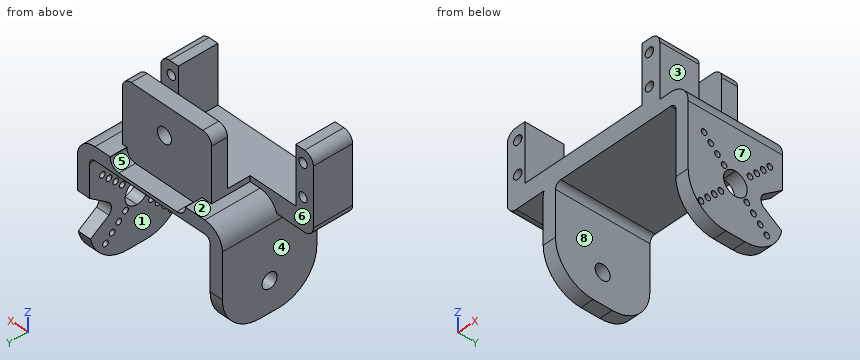
```python
from build123d import *

# Parameters (mm, degrees)
BOSS_EXTRUDE1_DEPTH     = 50
BOSS_EXTRUDE2_DEPTH     = 20.8
SKETCH4_W               = 50.8
SKETCH4_H               = 3
BOSS_EXTRUDE3_DEPTH     = 20.4
BOSS_EXTRUDE4_START     = 32.8
BOSS_EXTRUDE4_OUTLINE_W = 50.8
BOSS_EXTRUDE4_OUTLINE_H = 30.5
BOSS_EXTRUDE4_OUTLINE_R = 4
BOSS_EXTRUDE4_DEPTH     = 8.4
CUT_EXTRUDE1_OUTLINE_R  = 2.4
CUT_EXTRUDE1_DEPTH      = 20.8
FILLET1_R               = 5
FILLET2_R               = 20
SKETCH6_R               = 1.5
CUT_EXTRUDE2_DEPTH      = 28.4
CUT_EXTRUDE3_DEPTH      = 136.4
CUT_EXTRUDE4_DEPTH      = 132.215666798
CUT_EXTRUDE4_DEPTH_BACK = 26.4
CUT_EXTRUDE5_DEPTH      = 8.8


# Read off the part's stored shape, not the designer's step: Boss-Extrude4, Cut-Extrude1
with BuildPart() as part:
    # Sketch1 → Boss-Extrude1 (new body)
    with BuildSketch(Plane(origin=(0, 0, 0), x_dir=(1, 0, 0), z_dir=(0, 1, 0))):
        with BuildLine():
            Line((-56.375697839, 54.197981352), (-56.375697839, 10.497981352))
            ThreePointArc((-56.375697839, 10.497981352), (-53.44676565, 3.42691354), (-46.375697839, 0.497981352))
            Line((-46.375697839, 0.497981352), (16.224302161, 0.497981352))
            ThreePointArc((16.224302161, 0.497981352), (23.295369973, 3.42691354), (26.224302161, 10.497981352))
            Line((26.224302161, 10.497981352), (26.224302161, 64.097981352))
            Line((26.224302161, 64.097981352), (19.224302161, 64.097981352))
            Line((19.224302161, 64.097981352), (19.224302161, 10.497981352))
            ThreePointArc((19.224302161, 10.497981352), (18.345622505, 8.376661008), (16.224302161, 7.497981352))
            Line((16.224302161, 7.497981352), (-46.375697839, 7.497981352))
            ThreePointArc((-46.375697839, 7.497981352), (-48.497018182, 8.376661008), (-49.375697839, 10.497981352))
            Line((-49.375697839, 10.497981352), (-49.375697839, 54.197981352))
            Line((-49.375697839, 54.197981352), (-56.375697839, 54.197981352))
        make_face()
    extrude(amount=BOSS_EXTRUDE1_DEPTH)

    # Sketch2 → Boss-Extrude2 (add)
    with BuildSketch(Plane.XZ):
        with BuildLine():
            Line((-71.775697839, -7.497981352), (-55.915089853, -7.497981352))
            ThreePointArc((-55.915089853, -7.497981352), (-52.291777622, -2.435723603), (-46.375697839, -0.497981352))
            Line((-46.375697839, -0.497981352), (10.024302161, -0.497981352))
            Line((10.024302161, -0.497981352), (10.024302161, 33.002018648))
            Line((10.024302161, 33.002018648), (0.024302161, 33.002018648))
            Line((0.024302161, 33.002018648), (0.024302161, 2.502018648))
            Line((0.024302161, 2.502018648), (-66.775697839, 2.502018648))
            Line((-66.775697839, 2.502018648), (-66.775697839, 33.002018648))
            Line((-66.775697839, 33.002018648), (-76.775697839, 33.002018648))
            Line((-76.775697839, 33.002018648), (-76.775697839, -2.497981352))
            ThreePointArc((-76.775697839, -2.497981352), (-75.311231744, -6.033515257), (-71.775697839, -7.497981352))
        make_face()
    extrude(amount=-BOSS_EXTRUDE2_DEPTH)

    # Sketch4 → Boss-Extrude3 (add)
    with BuildSketch(Plane(origin=(0, 20.8, 0), x_dir=(1, 0, 0), z_dir=(0, 1, 0))):
        with Locations((-15.375697839, -1.002018648)):
            Rectangle(SKETCH4_W, SKETCH4_H)
    extrude(amount=BOSS_EXTRUDE3_DEPTH)

    # Boss-Extrude4 outline → Boss-Extrude4 (add)
    with BuildSketch(Plane(origin=(0, 0, 0), x_dir=(1, 0, 0), z_dir=(0, 1, 0)).offset(BOSS_EXTRUDE4_START)):
        with Locations((-15.375697839, -17.752018648)):
            Rectangle(BOSS_EXTRUDE4_OUTLINE_W, BOSS_EXTRUDE4_OUTLINE_H)
        with Locations((-13.903425018, -17.753309847)):
            Circle(BOSS_EXTRUDE4_OUTLINE_R, mode=Mode.SUBTRACT)
    extrude(amount=BOSS_EXTRUDE4_DEPTH)

    # Cut-Extrude1 outline → Cut-Extrude1 (cut)
    with BuildSketch(Plane(origin=(0, 0, 0), x_dir=(1, 0, 0), z_dir=(0, 1, 0))):
        with Locations((-70.875697839, -9.252018648)):
            Circle(CUT_EXTRUDE1_OUTLINE_R)
        with Locations((-70.875697839, -26.252018648)):
            Circle(CUT_EXTRUDE1_OUTLINE_R)
        with Locations((4.124302161, -26.252018648)):
            Circle(CUT_EXTRUDE1_OUTLINE_R)
        with Locations((4.124302161, -9.252018648)):
            Circle(CUT_EXTRUDE1_OUTLINE_R)
    extrude(amount=CUT_EXTRUDE1_DEPTH, mode=Mode.SUBTRACT)

    # Fillet1
    fillet1_edges = [part.edges().sort_by_distance(p)[0] for p in [
        (-76.775697839, 10.4, 33.002018648),
        (10.024302161, 10.4, 33.002018648),
        (10.024302161, 37, 33.002018648),
        (-40.775697839, 37, 33.002018648),
    ]]
    fillet(fillet1_edges, radius=FILLET1_R)

    # Fillet2
    fillet2_edges = [part.edges().sort_by_distance(p)[0] for p in [
        (22.724302161, 0, -64.097981352),
        (-52.875697839, 0, -54.197981352),
        (22.724302161, 50, -64.097981352),
        (-52.875697839, 50, -54.197981352),
    ]]
    fillet(fillet2_edges, radius=FILLET2_R)

    # Sketch6 → Cut-Extrude2 (cut)
    with BuildSketch(Plane(origin=(26.224302161, 0, 0), x_dir=(0, 0, -1), z_dir=(1, 0, 0))):
        with BuildLine():
            ThreePointArc((34.097981352, 25), (38.097981352, 21), (42.097981352, 25))
            Line((42.097981352, 25), (34.097981352, 25))
        make_face()
        with BuildLine():
            Line((34.097981352, 25), (42.097981352, 25))
            ThreePointArc((42.097981352, 25), (38.097981352, 29), (34.097981352, 25))
        make_face()
        with BuildLine():
            ThreePointArc((31.836343923, 25), (38.097981352, 18.738362572), (44.35961878, 25))
            Line((44.35961878, 25), (42.097981352, 25))
            ThreePointArc((42.097981352, 25), (38.097981352, 21), (34.097981352, 25))
            Line((34.097981352, 25), (31.836343923, 25))
        make_face()
        with BuildLine():
            Line((42.097981352, 25), (44.35961878, 25))
            ThreePointArc((44.35961878, 25), (38.097981352, 31.261637428), (31.836343923, 25))
            Line((31.836343923, 25), (34.097981352, 25))
            ThreePointArc((34.097981352, 25), (38.097981352, 29), (42.097981352, 25))
        make_face()
        with Locations((30.390517437, 32.707463915)):
            Circle(SKETCH6_R)
        with Locations((26.876196734, 36.221784617)):
            Circle(SKETCH6_R)
        with Locations((23.354804964, 39.743176388)):
            Circle(SKETCH6_R)
        with Locations((19.854626397, 43.243354955)):
            Circle(SKETCH6_R)
        with Locations((44.108388992, 31.01040764)):
            Circle(SKETCH6_R)
        with Locations((47.643922898, 34.545941546)):
            Circle(SKETCH6_R)
        with Locations((51.179456803, 38.081475452)):
            Circle(SKETCH6_R)
        with Locations((54.714990709, 41.617009358)):
            Circle(SKETCH6_R)
        with Locations((45.805445266, 17.292536085)):
            Circle(SKETCH6_R)
        with Locations((49.319765969, 13.778215383)):
            Circle(SKETCH6_R)
        with Locations((52.841157739, 10.256823612)):
            Circle(SKETCH6_R)
        with Locations((56.341336306, 6.756645045)):
            Circle(SKETCH6_R)
        with Locations((32.087573711, 18.98959236)):
            Circle(SKETCH6_R)
        with Locations((28.552039805, 15.454058454)):
            Circle(SKETCH6_R)
        with Locations((25.0165059, 11.918524548)):
            Circle(SKETCH6_R)
        with Locations((21.480971994, 8.382990642)):
            Circle(SKETCH6_R)
    extrude(amount=-CUT_EXTRUDE2_DEPTH, mode=Mode.SUBTRACT)

    # Sketch6<3> → Cut-Extrude3 (cut)
    with BuildSketch(Plane(origin=(26.224302161, 0, 0), x_dir=(0, 0, -1), z_dir=(1, 0, 0))):
        with BuildLine():
            ThreePointArc((34.097981352, 25), (38.097981352, 21), (42.097981352, 25))
            Line((42.097981352, 25), (34.097981352, 25))
        make_face()
        with BuildLine():
            Line((34.097981352, 25), (42.097981352, 25))
            ThreePointArc((42.097981352, 25), (38.097981352, 29), (34.097981352, 25))
        make_face()
    extrude(amount=-CUT_EXTRUDE3_DEPTH, mode=Mode.SUBTRACT)

    # Sketch7 → Cut-Extrude4 (cut, two sides: drawn at the far end of the back side and taken through both)
    with BuildSketch(Plane(origin=(26.224302161, 0, 0), x_dir=(0, 0, -1), z_dir=(1, 0, 0)).offset(-CUT_EXTRUDE4_DEPTH_BACK)):
        with BuildLine():
            Line((44.097981352, 50), (27.901409821, 50))
            Line((27.901409821, 50), (34.889942889, 40.363586132))
            ThreePointArc((34.889942889, 40.363586132), (38.136702541, 38.542544558), (41.629478365, 39.830239282))
            Line((41.629478365, 39.830239282), (48.26230961, 49.561655609))
            ThreePointArc((48.26230961, 49.561655609), (46.191648926, 49.890112018), (44.097981352, 50))
        make_face()
    extrude(amount=CUT_EXTRUDE4_DEPTH + CUT_EXTRUDE4_DEPTH_BACK, mode=Mode.SUBTRACT)

    # Sketch8 → Cut-Extrude5 (cut)
    with BuildSketch(Plane(origin=(0, 50, 0), x_dir=(1, 0, 0), z_dir=(0, 1, 0))):
        with BuildLine():
            Line((-35.363310125, -41.134391508), (7.556460089, -41.134391508))
            Line((7.556460089, -41.134391508), (7.556460089, 0.627771813))
            ThreePointArc((7.556460089, 0.627771813), (6.091993995, 4.163305719), (2.556460089, 5.627771813))
            Line((2.556460089, 5.627771813), (-30.363310125, 5.627771813))
            ThreePointArc((-30.363310125, 5.627771813), (-33.898844031, 4.163305719), (-35.363310125, 0.627771813))
            Line((-35.363310125, 0.627771813), (-35.363310125, -41.134391508))
        make_face()
    extrude(amount=-CUT_EXTRUDE5_DEPTH, mode=Mode.SUBTRACT)


solid = part.part
```
Here's how the part is built. I have some questions about the finished solid (model axes, mm). Face numbers are marked on the shaded views. A direction names the side the tool comes from. Give positions to 0.01 mm unless a question says otherwise; leave off trailing zeros. Write each loop counter-clockwise with the first axis right and the second up, starting at its lowest first coordinate (ties: lowest second). Pieces come first, ordered by that corner, then holes. Notation, with made-up numbers: (-27.75, 55.5) -> (8.25, 55.5) arc R26 cw to (8.25, 91.5) -> close; hole circle Ø4 at (-2.75, 89). An arc over 180 degrees is marked (long way). Use one line per item in the form item = value.
1) Suppose I cut it at D-D (x = 12). Please give me the cut outline in (y, z).
Verdict:
outline = (0, -7.5) -> (50, -7.5) -> (50, -0.5) -> (0, -0.5) -> close
2) If I drill on L1, parallel to X at y = 5, z = -41.5; L2, parallel to Y at x = 4, z = 14; L3, parallel to Z at x = -72, y = 12.5, over which ranges is the centre line in solid material (lowest first)? Write a range as [from, to].
Verdict:
L1 = [-56.38, -49.38], [19.22, 26.22]
L2 = [0, 20.8], [32.8, 41.2]
L3 = [-7.49, 7.13], [11.37, 24.13], [28.37, 33]
3) Suppose I cut it at A-A (x = -13). Please give me the cut outline in (y, z), and give its area (3 significant figures).
Verdict:
outline = (0, -7.5) -> (50, -7.5) -> (50, -5.63) -> (41.2, -5.63) -> (41.2, 13.86) -> (32.8, 13.86) -> (32.8, 2.5) -> (0, 2.5) -> close; (32.8, 21.65) -> (41.2, 21.65) -> (41.2, 33) -> (32.8, 33) -> close
area = 619 mm2
4) Suppose I cut it at B-B (x = -26). Please give me the cut outline in (y, z).
Verdict:
outline = (0, -7.5) -> (50, -7.5) -> (50, -5.63) -> (41.2, -5.63) -> (41.2, 33) -> (32.8, 33) -> (32.8, 2.5) -> (0, 2.5) -> close
5) I'm going to push flat-ended pins straight in: pin 1 (1 mm diameter, centred on x = -13, y = 28.5, fed in from +Z); pin 2 (3 mm diameter, centred on x = 7, z = 18.5, fed in from +Y); pin 3 (16.5 mm diameter, centred on y = 12, z = 20, fed in from +X). Where does each tip first touch, or does it pass through?
Verdict:
pin_1 = 2.5
pin_2 = 41.2
pin_3 = 10.02
6) On a 3-axis mill with a long thin cutter (end or side, diameter ignored), from which of +Z, -Z, +X, -X, +Y, -Y can I reach the whole of each face in a straight line? I mean the marked faces 1, 2, 3, 4 and 5. Say none if no direction works.
Verdict:
face_1 = -Z, +Y, -Y
face_2 = +Z, -X, +Y
face_3 = +Z, +X, +Y, -Y
face_4 = -Z, -X, +Y, -Y
face_5 = +Z, +Y
7) Suppose I cut it at C-C (x = -60.5). Please give me the cut outline in (y, z).
Verdict:
outline = (0, -7.5) -> (20.8, -7.5) -> (20.8, 2.5) -> (0, 2.5) -> close
8) We'd pull the mould along X, two halves only. Please class the marked faces 6, 7 and 8: +X half, -X half, draft (parallel to the pull), parting line (faces both ways), or undercut.
Verdict:
face_6 = draft
face_7 = +X half
face_8 = undercut
